from build123d import *

# Parameters (mm, degrees)
F0_W     = 15
F0_H     = 10
F1_DEPTH = 10
F2_R     = 3
F3_DEPTH = 15.8
F5_DEPTH = 5
F6_R     = 5
F6_R_2   = 3
F7_DEPTH = 2


with BuildPart() as f1:
    # F0 (on Front) → F1 (new body)
    with BuildSketch(Plane.XZ):
        Polygon((-10, 0), (0, 0), (0, 10), (0, 30), (0, 40), (-10, 40), align=None)
        with Locations((7.5, 5)):
            Rectangle(F0_W, F0_H)
        with Locations((7.5, 35)):
            Rectangle(F0_W, F0_H)
    extrude(amount=F1_DEPTH)

    # F2 (on face) → F3 (join, symmetric)
    with BuildSketch(Plane(origin=(0, 0, 0), x_dir=(1, 0, 0), z_dir=(0, 0, -1))):
        with Locations((8.7596364319, 5)):
            Circle(F2_R)
    extrude(amount=F3_DEPTH, both=True)

    # F4 (on face) → F5 (join)
    with BuildSketch(Plane(origin=(0, 0, -15.8), x_dir=(1, 0, 0), z_dir=(0, 0, -1))):
        with BuildLine():
            Line((-3.7403635681, 2), (8.7596364319, 2))
            ThreePointArc((8.7596364319, 2), (5.7596364319, 5), (8.7596364319, 8))
            Line((8.7596364319, 8), (-3.7403635681, 8))
            Line((-3.7403635681, 8), (-3.7403635681, 2))
        make_face()
        with BuildLine():
            Line((8.7596364319, 2), (21.2596364319, 2))
            Line((21.2596364319, 2), (21.2596364319, 8))
            Line((21.2596364319, 8), (8.7596364319, 8))
            ThreePointArc((8.7596364319, 8), (10.8809567755, 7.1213203436), (11.7596364319, 5))
            ThreePointArc((11.7596364319, 5), (10.8809567755, 2.8786796564), (8.7596364319, 2))
        make_face()
        with BuildLine():
            ThreePointArc((8.7596364319, 8), (5.7596364319, 5), (8.7596364319, 2))
            ThreePointArc((8.7596364319, 2), (10.8809567755, 2.8786796564), (11.7596364319, 5))
            ThreePointArc((11.7596364319, 5), (10.8809567755, 7.1213203436), (8.7596364319, 8))
        make_face()
    extrude(amount=F5_DEPTH)

    # F6 (on face) → F7 (join)
    with BuildSketch(Plane.XY.offset(15.8)):
        with Locations((8.7596364319, -5)):
            Circle(F6_R)
        with Locations((8.7596364319, -5)):
            Circle(F6_R_2, mode=Mode.SUBTRACT)
        with Locations((8.7596364319, -5)):
            Circle(F6_R_2)
    extrude(amount=F7_DEPTH)


solid = f1.part
The listing builds one solid part. Answer for the finished solid, in the listing's coordinates (mm). A direction names the side the tool comes from. Give positions to 0.01 mm unless a question says otherwise; leave off trailing zeros. Write each loop counter-clockwise with the first axis right and the second up, starting at its lowest first coordinate (ties: lowest second). Pieces come first, ordered by that corner, then holes.
Item 1: Which of the six approach directions +Z, -Z, +X, -X, +Y, -Y give full straight-line access (tool end or side, diameter ignored) to faces 1 (the cylindrical face through (13.378, -6.915, 16.786)), 2 (the flat face through (-3.74, -5, -18)), 3 (the flat face through (9, -2, -18))?
Item 2: Determine the mould class of faces 4 (the flat face through (15, -5, 35)), 5 (the cylindrical face through (10.144, -2.338, 12.859)), 6 (the flat face through (9, -5, -20.8)), 7 (the flat face through (3, -5, 40)) for opening direction Z: released by +Z, released by -Z, zero draft, split by the parting line, or undercut.
Item 3: Section A-A, the plane x = 9.5 is taken. Write down the section's boundary in (y, z), plus the area to 3 significant figures.
Item 4: Flat-ended cylindrical pins translate along their axes: P1, Ø5, axis at y = -4.5, z = -1, coming from the +X side; P2, Ø1.8, axis at x = 18, y = -5, coming from the +Z side; P3, Ø1, axis at y = -9, z = -11.5, coming from the +X side; P4, Ø2.5, axis at y = -4.5, z = -19, coming from the -X side. Find the tip coordinate at first contact, or state that the pin passes through.
Item 5: Find the intervals of material crossed by line 1 along Z through (x, y) = (2, -7); line 2 along Z through (x, y) = (7.5, -0.5); line 3 along Z through (x, y) = (-3, -4.5), in increasing order.
Item 6: Section B-B, the plane y = -5 is taken. Write down the section's boundary in (x, z).
Item 7: Section C-C, the plane y = -8.75 is taken. Write down the section's boundary in (x, z).
Item 8: Section D-D, the plane z = -15 is taken. Write down the section's boundary in (x, y).
Completed:
1. face 1: none
1. face 2: -Z, -X, +Y, -Y
1. face 3: -Z, +X, -X, +Y
2. face 4: zero draft
2. face 5: undercut
2. face 6: released by -Z
2. face 7: released by +Z
3. outline: (-10, 0) - (-7.91, 0) - (-7.91, -15.8) - (-8, -15.8) - (-8, -20.8) - (-2, -20.8) - (-2, -15.8) - (-2.09, -15.8) - (-2.09, 0) - (0, 0) - (0, 10) - (-2.09, 10) - (-2.09, 15.8) - (-0.06, 15.8) - (-0.06, 17.8) - (-9.94, 17.8) - (-9.94, 15.8) - (-7.91, 15.8) - (-7.91, 10) - (-10, 10) - close; (-10, 30) - (0, 30) - (0, 40) - (-10, 40) - close
3. area: 375 mm2
4. P1: stops at x = 15
4. P2: stops at z = -15.8
4. P3: passes through
4. P4: stops at x = -3.74
5. line 1: z = -20.8 to -15.8, 0 to 10, 30 to 40
5. line 2: z = 0 to 10, 15.8 to 17.8, 30 to 40
5. line 3: z = -20.8 to -15.8, 0 to 40
6. outline: (-10, 0) - (5.76, 0) - (5.76, -15.8) - (-3.74, -15.8) - (-3.74, -20.8) - (21.26, -20.8) - (21.26, -15.8) - (11.76, -15.8) - (11.76, 0) - (15, 0) - (15, 10) - (11.76, 10) - (11.76, 15.8) - (13.76, 15.8) - (13.76, 17.8) - (3.76, 17.8) - (3.76, 15.8) - (5.76, 15.8) - (5.76, 10) - (0, 10) - (0, 30) - (15, 30) - (15, 40) - (-10, 40) - close
7. outline: (-10, 0) - (15, 0) - (15, 10) - (0, 10) - (0, 30) - (15, 30) - (15, 40) - (-10, 40) - close; (5.45, 15.8) - (12.07, 15.8) - (12.07, 17.8) - (5.45, 17.8) - close
8. outline: circle Ø6 at (8.76, -5)
